from build123d import *

# Parameters (mm, degrees)
EXTRUDE_1_DEPTH     = 9
SKETCH_2_R          = 3.25
CUT_EXTRUDE_1_DEPTH = 9
SKETCH_3_R          = 3.25
CUT_EXTRUDE_2_DEPTH = 9


with BuildPart() as part:
    # Эскиз1 → Бобышка-Вытянуть1 (new body, symmetric)
    with BuildSketch(Plane.XY):
        Polygon((-50, 0), (0, 0), (0, 50), (-8, 50), (-8, 40.5), (-7.5, 40), (-8, 39.5), (-8, 28), (-28, 8), (-39.5, 8), (-40, 7.5), (-40.5, 8), (-50, 8), align=None)
        with BuildLine():
            Line((-4.5, 12), (-4.5, 24.560303038))
            ThreePointArc((-4.5, 24.560303038), (-5.117316568, 25.484182571), (-6.207106781, 25.267409819))
            Line((-6.207106781, 25.267409819), (-25.267409819, 6.207106781))
            ThreePointArc((-25.267409819, 6.207106781), (-25.484182571, 5.117316568), (-24.560303038, 4.5))
            Line((-24.560303038, 4.5), (-12, 4.5))
            Line((-12, 4.5), (-12, 7.9))
            ThreePointArc((-12, 7.9), (-14.899137803, 9.100862197), (-16.1, 12))
            ThreePointArc((-16.1, 12), (-15.1, 13), (-14.1, 12))
            ThreePointArc((-14.1, 12), (-10.51507576, 10.51507576), (-12, 14.1))
            ThreePointArc((-12, 14.1), (-13, 15.1), (-12, 16.1))
            ThreePointArc((-12, 16.1), (-9.100862197, 14.899137803), (-7.9, 12))
            Line((-7.9, 12), (-4.5, 12))
        make_face(mode=Mode.SUBTRACT)
    extrude(amount=EXTRUDE_1_DEPTH, both=True)

    # Эскиз2 → Вырез-Вытянуть1 (cut, through all)
    with BuildSketch(Plane.ZY.offset(8)):
        with Locations(Location((0, 40, 0), (0, 0, 270))):  # turned: the seam where the file's is
            Circle(SKETCH_2_R)
    extrude(amount=-CUT_EXTRUDE_1_DEPTH, mode=Mode.SUBTRACT)

    # Эскиз3 → Вырез-Вытянуть2 (cut, through all)
    with BuildSketch(Plane(origin=(0, 8, 0), x_dir=(1, 0, 0), z_dir=(0, 1, 0))):
        with Locations(Location((-40, 0, 0), (0, 0, 180))):  # turned: the seam where the file's is
            Circle(SKETCH_3_R)
    extrude(amount=-CUT_EXTRUDE_2_DEPTH, mode=Mode.SUBTRACT)


solid = part.part
For this review, take the finished solid that the model builds, in its own axes (mm). A direction names the side the tool comes from. Give positions to 0.01 mm unless a question says otherwise; leave off trailing zeros. Order: outer loops, then holes, each group sorted by start corner. A loop starts at its lowest first (then second) coordinate and runs counter-clockwise, first axis right, second up. Notation, with made-up numbers: (-5.75, 77) - (29.25, 77) arc R11 cw to (29.25, 81) - close; hole circle Ø7 at (-12.5, 16.25). An arc over 180 degrees is marked (long way). Answer as a JSON object with one key per item and string values. Group by question number.
Item 1: Machinability: for faces 4 (the flat face through (0, 25, 0)), 5 (the flat face through (-45, 8, 0)), 6 (the flat face through (-18, 4.5, 0)), which of the approach directions +Z, -Z, +X, -X, +Y, -Y give a long, thin tool a straight path to every point of the face, cutting with its end or side? Answer none if there is none.
Item 2: Take a section at C-C on x = -17. Give the boundary of the cut face in (y, z).
Item 3: Draft analysis for pull direction X (two halves, no side actions). For faces 1 (the flat face through (-6, 12, 0)), 2 (the flat face through (-16, 18, 9)), 3 (the flat face through (-8, 34, 0)), state which applies: pulls with the +X half, pulls with the -X half, needs draft (parallel to the pull), parting line crosses it, or undercut.
Item 4: Take a section at B-B on y = 11. Give the boundary of the cut face in (x, z), and give its area (3 significant figures).
Item 5: Take a section at D-D on z = -4.5. Give the boundary of the cut face in (x, y), and give its area (3 significant figures).
Item 6: Clearance check with flat-ended pins moving along their axes: pin 1 Ø9 at (y, z) = (35.5, -4) entering from -X; pin 2 Ø5 at (x, z) = (-47, -4) entering from +Y; pin 3 Ø4 at (x, z) = (-19.5, -3) entering from +Y; pin 4 Ø3.5 at (x, y) = (-12, 12) entering from -Z. State where each tip first meets the part, or that it passes through.
Item 7: Wall thickness on line 1 along Z through (x, y) = (-2, 40); line 2 along Y through (x, z) = (-2.5, 0); line 3 along X through (y, z) = (12.5, 6.25): over which ranges is each line inside the solid? List them lowest first.
Item 8: Take a section at A-A on z = 0. Give the boundary of the cut face in (x, y).
Reported:
{
 "1": {"face 4": "+Z, -Z, +X, +Y, -Y", "face 5": "+Z, -Z, -X, +Y", "face 6": "+Z, -Z"},
 "2": {"outline": "(0, -9) - (4.5, -9) - (4.5, 9) - (0, 9) - close; (14.47, -9) - (19, -9) - (19, 9) - (14.47, 9) - close"},
 "3": {"face 1": "undercut", "face 2": "needs draft", "face 3": "pulls with the -X half"},
 "4": {"outline": "(-25, -9) - (-20.47, -9) - (-20.47, 9) - (-25, 9) - close; (-15.98, -9) - (-13.85, -9) - (-13.85, 9) - (-15.98, 9) - close; (-10.15, -9) - (0, -9) - (0, 9) - (-10.15, 9) - close", "area": "303 mm^2"},
 "5": {"outline": "(-50, 0) - (0, 0) - (0, 50) - (-8, 50) - (-8, 40.5) - (-7.5, 40) - (-8, 39.5) - (-8, 28) - (-28, 8) - (-39.5, 8) - (-40, 7.5) - (-40.5, 8) - (-50, 8) - close; hole (-25.27, 6.21) arc R1 ccw to (-24.56, 4.5) - (-12, 4.5) - (-12, 7.9) arc R4.1 cw to (-16.1, 12) arc R1 cw to (-14.1, 12) arc R2.1 ccw (long way) to (-12, 14.1) arc R1 cw to (-12, 16.1) arc R4.1 cw to (-7.9, 12) - (-4.5, 12) - (-4.5, 24.56) arc R1 ccw to (-6.21, 25.27) - close", "area": "761 mm^2"},
 "6": {"pin 1": "x = -8", "pin 2": "y = 8", "pin 3": "y = 18.5", "pin 4": "through"},
 "7": {"line 1": "-9 to -3.25, 3.25 to 9", "line 2": "0 to 36.75, 43.25 to 50", "line 3": "-23.5 to -18.97, -15.97 to -14.23, -9.96 to -7.93, -4.5 to 0"},
 "8": {"outline": "(-50, 0) - (-43.25, 0) - (-43.25, 8) - (-50, 8) - close; (-36.75, 0) - (0, 0) - (0, 36.75) - (-8, 36.75) - (-8, 28) - (-28, 8) - (-36.75, 8) - close; (-8, 43.25) - (0, 43.25) - (0, 50) - (-8, 50) - close; hole (-25.27, 6.21) arc R1 ccw to (-24.56, 4.5) - (-12, 4.5) - (-12, 7.9) arc R4.1 cw to (-16.1, 12) arc R1 cw to (-14.1, 12) arc R2.1 ccw (long way) to (-12, 14.1) arc R1 cw to (-12, 16.1) arc R4.1 cw to (-7.9, 12) - (-4.5, 12) - (-4.5, 24.56) arc R1 ccw to (-6.21, 25.27) - close"}
}
